Part model, mm, in its own coordinate system. Coordinates: 2 decimals unless noted, no trailing zeros. Loops run counter-clockwise (first coordinate to the right, second up) from the corner with the lowest first, then second, coordinate; pieces in that order, holes last.
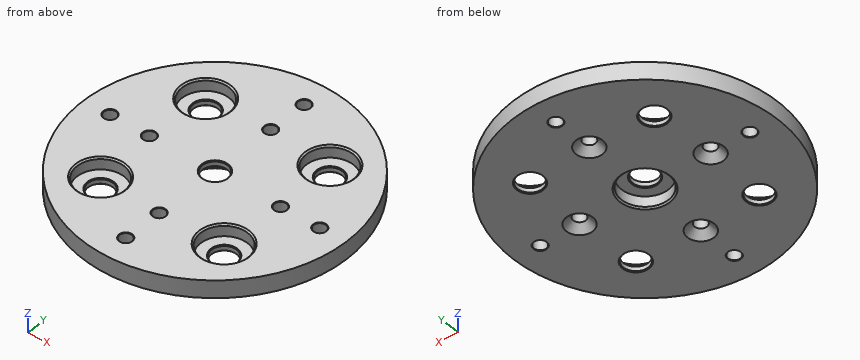
```python
from build123d import *

# Parameters (mm, degrees)
SKETCH1_R                                      = 90
BOSS_EXTRUDE1_DEPTH                            = 12
CBORE_FOR_M5_HEX_HEAD_BOLT1_AT_2_COUNT         = 2
CBORE_FOR_M5_HEX_HEAD_BOLT1_AT_2_PITCH         = 85.093412723
CBORE_FOR_M5_HEX_HEAD_BOLT1_AT_3_COUNT         = 2
CBORE_FOR_M5_HEX_HEAD_BOLT1_AT_3_PITCH         = 120.339778661
CBORE_FOR_M5_HEX_HEAD_BOLT1_AT_4_COUNT         = 2
CBORE_FOR_M5_HEX_HEAD_BOLT1_AT_4_PITCH         = 85.093412723
CSK_FOR_M5_FLAT_HEAD_MACHINE_SCREW1_AT_2_COUNT = 2
CSK_FOR_M5_FLAT_HEAD_MACHINE_SCREW1_AT_2_PITCH = 63.63491592
CSK_FOR_M5_FLAT_HEAD_MACHINE_SCREW1_AT_3_COUNT = 2
CSK_FOR_M5_FLAT_HEAD_MACHINE_SCREW1_AT_3_PITCH = 89.995540664
CSK_FOR_M5_FLAT_HEAD_MACHINE_SCREW1_AT_4_COUNT = 2
CSK_FOR_M5_FLAT_HEAD_MACHINE_SCREW1_AT_4_PITCH = 63.627500237
CSK_FOR_M5_FLAT_HEAD_MACHINE_SCREW2_AT_2_COUNT = 2
CSK_FOR_M5_FLAT_HEAD_MACHINE_SCREW2_AT_2_PITCH = 101.823376491
CSK_FOR_M5_FLAT_HEAD_MACHINE_SCREW2_AT_3_COUNT = 2
CSK_FOR_M5_FLAT_HEAD_MACHINE_SCREW2_AT_3_PITCH = 144
CSK_FOR_M5_FLAT_HEAD_MACHINE_SCREW2_AT_4_COUNT = 2
CSK_FOR_M5_FLAT_HEAD_MACHINE_SCREW2_AT_4_PITCH = 101.823376491


with BuildPart() as part:
    # Sketch1 → Boss-Extrude1 (new body)
    with BuildSketch(Plane.XY):
        Circle(SKETCH1_R)
    extrude(amount=BOSS_EXTRUDE1_DEPTH)

    # Sketch4 → CBORE for M5 Hex Head Bolt1 (revolve, cut)
    with BuildSketch(Plane(origin=(42.666666667, 42.666666667, 12), x_dir=(0, -1, 0), z_dir=(1, 0, 0))):
        Polygon((0, 0), (0, 12), (9, 12), (8.5, 11.5), (8.5, 8.5), (9, 8), (16, 8), (16, 1), (17, 0), align=None)
    cbore_for_m5_hex_head_bolt1 = revolve(axis=Axis((42.666666667, 42.666666667, 18.35), (0, 0, -1)), mode=Mode.SUBTRACT)

    # CBORE for M5 Hex Head Bolt1 at 2: CBORE for M5 Hex Head Bolt1 ×2
    with Locations(*[Vector(-0.0028234828970208348, -0.9999960139642209, 0) * (i * CBORE_FOR_M5_HEX_HEAD_BOLT1_AT_2_PITCH) for i in range(1, CBORE_FOR_M5_HEX_HEAD_BOLT1_AT_2_COUNT)]):
        add(cbore_for_m5_hex_head_bolt1, mode=Mode.SUBTRACT)

    # CBORE for M5 Hex Head Bolt1 at 3: CBORE for M5 Hex Head Bolt1 ×2
    with Locations(*[Vector(-0.7071067811865486, -0.7071067811865465, 0) * (i * CBORE_FOR_M5_HEX_HEAD_BOLT1_AT_3_PITCH) for i in range(1, CBORE_FOR_M5_HEX_HEAD_BOLT1_AT_3_COUNT)]):
        add(cbore_for_m5_hex_head_bolt1, mode=Mode.SUBTRACT)

    # CBORE for M5 Hex Head Bolt1 at 4: CBORE for M5 Hex Head Bolt1 ×2
    with Locations(*[Vector(-0.9999960139642209, -0.002823482897031568, 0) * (i * CBORE_FOR_M5_HEX_HEAD_BOLT1_AT_4_PITCH) for i in range(1, CBORE_FOR_M5_HEX_HEAD_BOLT1_AT_4_COUNT)]):
        add(cbore_for_m5_hex_head_bolt1, mode=Mode.SUBTRACT)

    # Sketch5 → CBORE for M5 Hex Head Bolt2 (revolve, cut)
    with BuildSketch(Plane.YZ):
        Polygon((0, 0), (0, 12), (9, 12), (8.5, 11.5), (8.5, 8.5), (9, 8), (16, 8), (16, 1), (17, 0), align=None)
    revolve(axis=Axis((0, 0, -6.35), (0, 0, 1)), mode=Mode.SUBTRACT)

    # Sketch6 → CSK for M5 Flat Head Machine Screw1 (revolve, cut)
    with BuildSketch(Plane(origin=(44.991952442, -0.003388792, 0), x_dir=(0, 1, 0), z_dir=(1, 0, 0))):
        Polygon((0, 0), (0, 12), (4.5, 12), (4.2, 11.7), (4.2, 4.8), (9, 0), align=None)
    csk_for_m5_flat_head_machine_screw1 = revolve(axis=Axis((44.991952442, -0.003388792, -6.35), (0, 0, 1)), mode=Mode.SUBTRACT)

    # CSK for M5 Flat Head Machine Screw1 at 2: CSK for M5 Flat Head Machine Screw1 ×2
    with Locations(*[Vector(-0.7070545332830015, 0.7071590252297972, 0) * (i * CSK_FOR_M5_FLAT_HEAD_MACHINE_SCREW1_AT_2_PITCH) for i in range(1, CSK_FOR_M5_FLAT_HEAD_MACHINE_SCREW1_AT_2_COUNT)]):
        add(csk_for_m5_flat_head_machine_screw1, mode=Mode.SUBTRACT)

    # CSK for M5 Flat Head Machine Screw1 at 3: CSK for M5 Flat Head Machine Screw1 ×2
    with Locations(*[Vector(-0.9999999985437752, 5.396711723824618e-05, 0) * (i * CSK_FOR_M5_FLAT_HEAD_MACHINE_SCREW1_AT_3_PITCH) for i in range(1, CSK_FOR_M5_FLAT_HEAD_MACHINE_SCREW1_AT_3_COUNT)]):
        add(csk_for_m5_flat_head_machine_screw1, mode=Mode.SUBTRACT)

    # CSK for M5 Flat Head Machine Screw1 at 4: CSK for M5 Flat Head Machine Screw1 ×2
    with Locations(*[Vector(-0.707086531592279, -0.7071270302009401, 0) * (i * CSK_FOR_M5_FLAT_HEAD_MACHINE_SCREW1_AT_4_PITCH) for i in range(1, CSK_FOR_M5_FLAT_HEAD_MACHINE_SCREW1_AT_4_COUNT)]):
        add(csk_for_m5_flat_head_machine_screw1, mode=Mode.SUBTRACT)

    # Sketch8 → CSK for M5 Flat Head Machine Screw2 (revolve, cut)
    with BuildSketch(Plane(origin=(-72, 0, 12), x_dir=(0, -1, 0), z_dir=(1, 0, 0))):
        Polygon((0, 0), (0, 12), (4.5, 12), (4.2, 11.7), (4.2, 0.3), (4.5, 0), align=None)
    csk_for_m5_flat_head_machine_screw2 = revolve(axis=Axis((-72, 0, 18.35), (0, 0, -1)), mode=Mode.SUBTRACT)

    # CSK for M5 Flat Head Machine Screw2 at 2: CSK for M5 Flat Head Machine Screw2 ×2
    with Locations(*[Vector(0.7071067811865477, 0.7071067811865474, 0) * (i * CSK_FOR_M5_FLAT_HEAD_MACHINE_SCREW2_AT_2_PITCH) for i in range(1, CSK_FOR_M5_FLAT_HEAD_MACHINE_SCREW2_AT_2_COUNT)]):
        add(csk_for_m5_flat_head_machine_screw2, mode=Mode.SUBTRACT)

    # CSK for M5 Flat Head Machine Screw2 at 3: CSK for M5 Flat Head Machine Screw2 ×2
    with Locations(*[(i * CSK_FOR_M5_FLAT_HEAD_MACHINE_SCREW2_AT_3_PITCH, 0, 0) for i in range(1, CSK_FOR_M5_FLAT_HEAD_MACHINE_SCREW2_AT_3_COUNT)]):
        add(csk_for_m5_flat_head_machine_screw2, mode=Mode.SUBTRACT)

    # CSK for M5 Flat Head Machine Screw2 at 4: CSK for M5 Flat Head Machine Screw2 ×2
    with Locations(*[Vector(0.7071067811865475, -0.7071067811865476, 0) * (i * CSK_FOR_M5_FLAT_HEAD_MACHINE_SCREW2_AT_4_PITCH) for i in range(1, CSK_FOR_M5_FLAT_HEAD_MACHINE_SCREW2_AT_4_COUNT)]):
        add(csk_for_m5_flat_head_machine_screw2, mode=Mode.SUBTRACT)


solid = part.part
```
Q1. Drop flat-ended pins along their axis: P1, Ø1.5, axis at y = -36.5, z = 7.5, coming from the +X side (3 decimals); P2, Ø9.5, axis at x = 36.5, y = 41.5, coming from the +Z side; P3, Ø2, axis at x = 63, z = 3.5, coming from the -Y side. Give the stop position or say it passes through.
Q2. Saw through at C-C (y = -20). List the corners of the cut face in (x, z), plus the area to 3 significant figures.
Q3. Probe line 1 (X direction, y = -5.5, z = 3); line 2 (Y direction, x = 54.5, z = 9); line 3 (X direction, y = -33.5, z = 9.75). List the from-to ranges inside material, lowest first.
Q4. Saw through at A-A (y = 72). List the corners of the cut face in (x, z).
Checked values:
1. P1: stops at x = 82.595
1. P2: stops at z = 4
1. P3: stops at y = -65.24
2. outline: (-87.75, 0) - (87.75, 0) - (87.75, 12) - (-87.75, 12) - close
2. area: 2,110 mm2
3. line 1: x = -89.83 to -47.4, -42.61 to -15.02, 15.02 to 42.59, 47.4 to 89.83
3. line 2: y = -71.62 to -52.93, -31.93 to 31.9, 53.44 to 71.62
3. line 3: x = -83.53 to -55.7, -29.15 to 29.15, 55.7 to 83.53
4. outline: (-54, 0) - (-4.5, 0) - (-4.2, 0.3) - (-4.2, 11.7) - (-4.5, 12) - (-54, 12) - close; (4.2, 0.3) - (4.5, 0) - (54, 0) - (54, 12) - (4.5, 12) - (4.2, 11.7) - close
